For this review, take the finished solid that the model builds, in its own axes (mm). A direction names the side the tool comes from. Round coordinates to 2 decimals unless told otherwise and drop trailing zeros. Write each loop counter-clockwise with the first axis right and the second up, starting at its lowest first coordinate (ties: lowest second). Pieces come first, ordered by that corner, then holes. Notation, with made-up numbers: (-12.75, 0.5) -> (6.25, 0.5) arc R16 ccw to (6.25, 30.5) -> close; hole circle Ø1 at (88, 33). An arc over 180 degrees is marked (long way). Answer in a Markdown table with one row per item. Add a question column.
```python
from build123d import *

# Parameters (mm, degrees)
SKETCH1_W           = 610
SKETCH1_H           = 406
BOSS_EXTRUDE1_DEPTH = 11.1125
SKETCH3_W           = 120.65
SKETCH3_H           = 32.62
CUT_EXTRUDE2_DEPTH  = 367.548070048
SKETCH8_W           = 76.2
SKETCH8_H           = 32.62
CUT_EXTRUDE3_DEPTH  = 367.548070048
SKETCH4_R           = 3.3782
CUT_EXTRUDE4_DEPTH  = 367.548070048


with BuildPart() as part:
    # Sketch1 → Boss-Extrude1 (new body)
    with BuildSketch(Plane(origin=(0, 0, 0), x_dir=(0, 0, -1), z_dir=(1, 0, 0))):
        Rectangle(SKETCH1_W, SKETCH1_H)
    extrude(amount=BOSS_EXTRUDE1_DEPTH)

    # Sketch3 → Cut-Extrude2 (cut, through all)
    with BuildSketch(Plane(origin=(11.1125, 0, 0), x_dir=(0, 0, -1), z_dir=(1, 0, 0))):
        with Locations((203.4, 186.69)):
            Rectangle(SKETCH3_W, SKETCH3_H)
    cut_extrude2 = extrude(amount=-CUT_EXTRUDE2_DEPTH, mode=Mode.SUBTRACT)

    # Sketch8 → Cut-Extrude3 (cut, through all)
    with BuildSketch(Plane(origin=(11.1125, 0, 0), x_dir=(0, 0, -1), z_dir=(1, 0, 0))):
        with Locations((-192.086299996, 186.69)):
            Rectangle(SKETCH8_W, SKETCH8_H)
    cut_extrude3 = extrude(amount=-CUT_EXTRUDE3_DEPTH, mode=Mode.SUBTRACT)

    # Mirror3: Cut-Extrude2, Cut-Extrude3 across plane
    add(cut_extrude2.mirror(Plane.ZX), mode=Mode.SUBTRACT)
    add(cut_extrude3.mirror(Plane.ZX), mode=Mode.SUBTRACT)

    # Sketch4 → Cut-Extrude4 (cut, through all)
    with BuildSketch(Plane(origin=(11.1125, 0, 0), x_dir=(0, 0, -1), z_dir=(1, 0, 0))):
        with Locations(Location((-292.5, 165.50000007, 0), (0, 0, 90))):
            Circle(SKETCH4_R)
        with Locations(Location((-292.5, 55.16666669, 0), (0, 0, 90))):
            Circle(SKETCH4_R)
        with Locations(Location((-292.5, -55.16666669, 0), (0, 0, 90))):
            Circle(SKETCH4_R)
        with Locations(Location((-292.5, -165.50000007, 0), (0, 0, 90))):
            Circle(SKETCH4_R)
        with Locations(Location((292.5, -165.50000007, 0), (0, 0, 270))):
            Circle(SKETCH4_R)
        with Locations(Location((292.5, -55.16666669, 0), (0, 0, 270))):
            Circle(SKETCH4_R)
        with Locations(Location((292.5, 165.50000007, 0), (0, 0, 270))):
            Circle(SKETCH4_R)
        with Locations(Location((292.5, 55.16666669, 0), (0, 0, 270))):
            Circle(SKETCH4_R)
        with Locations(Location((-267.50000007, 190.5, 0), (0, 0, 90))):
            Circle(SKETCH4_R)
        with Locations(Location((-115.886299996, 190.5, 0), (0, 0, 90))):
            Circle(SKETCH4_R)
        with Locations(Location((-42.265866664, 190.5, 0), (0, 0, 90))):
            Circle(SKETCH4_R)
        with Locations(Location((31.354566668, 190.5, 0), (0, 0, 90))):
            Circle(SKETCH4_R)
        with Locations(Location((104.975, 190.5, 0), (0, 0, 90))):
            Circle(SKETCH4_R)
        with Locations(Location((104.975, -190.5, 0), (0, 0, 270))):
            Circle(SKETCH4_R)
        with Locations(Location((31.354566668, -190.5, 0), (0, 0, 270))):
            Circle(SKETCH4_R)
        with Locations(Location((-42.265866664, -190.5, 0), (0, 0, 270))):
            Circle(SKETCH4_R)
        with Locations(Location((-115.886299996, -190.5, 0), (0, 0, 270))):
            Circle(SKETCH4_R)
        with Locations(Location((-267.50000007, -190.5, 0), (0, 0, 270))):
            Circle(SKETCH4_R)
    extrude(amount=-CUT_EXTRUDE4_DEPTH, mode=Mode.SUBTRACT)


solid = part.part
```
1. The part is to be moulded in two halves that separate along Z. For faces 4 (the flat face through (5, -3, -305)), 5 (the flat face through (5, -3, 305)), 6 (the flat face through (6, 186, -143.075)), 7 (the flat face through (5, 203, 268)), say which applies: pulls with the +Z half, pulls with the -Z half, needs draft (parallel to the pull), parting line crosses it, or undercut.
2. Clearance check with flat-ended pins moving along their axes: pin 1 Ø6 at (y, z) = (-190.5, 115.89) entering from -X; pin 2 Ø5.5 at (x, z) = (5, -233) entering from +Y; pin 3 Ø5.5 at (x, z) = (6.5, 210) entering from -Y. State where each tip first meets the part, or that it passes through.
3. Tool access review of faces 1 (the flat face through (6, -186, 153.986)), 2 (the flat face through (6, 186, -263.725)), 3 (the flat face through (5, 203, 8)): name each direction out of +Z, -Z, +X, -X, +Y, -Y from which nothing blocks a thin tool from reaching the whole face with its end or side.
4. We need section B-B (x = 5.25). Count the separate pieces of the cut face and the enclosed holes in it, plus the area to 3 significant figures.
5. For L1, parallel to Y at x = 3.25, z = -292.5; L2, parallel to Z at x = 8, y = 165.5; L3, parallel to Z at x = 10, y = -187 (3 decimals), list the stretches that pass through material, from the lowest coordinate up. Write a range as [from, to].
6. We need section A-A (z = -168). Write out the cut boundary in (x, y).
Response:
| question | item | result |
|---|---|---|
| 1 | face 4 | pulls with the -Z half |
| 1 | face 5 | pulls with the +Z half |
| 1 | face 6 | undercut |
| 1 | face 7 | needs draft |
| 2 | pin 1 | through |
| 2 | pin 2 | y = 170.38 |
| 2 | pin 3 | y = -170.38 |
| 3 | face 1 | +X, -X, -Y |
| 3 | face 2 | +X, -X, +Y |
| 3 | face 3 | +Z, -Z, +X, -X, +Y |
| 4 | separate pieces | 1 |
| 4 | enclosed holes | 18 |
| 4 | area | 234,000 mm2 |
| 5 | L1 | [-203, -168.88], [-162.12, -58.54], [-51.79, 51.79], [58.54, 162.12], [168.88, 203] |
| 5 | L2 | [-305, -295.88], [-289.12, 289.12], [295.88, 305] |
| 5 | L3 | [-305, -263.725], [-143.075, 153.986], [230.186, 305] |
| 6 | outline | (0, -170.38) -> (11.11, -170.38) -> (11.11, 170.38) -> (0, 170.38) -> close |
